Could you check a few things on this drawing? It's one solid part, dimensions in mm from its lowest x, y, z. A direction names the side the tool comes from. Give positions to 0.01 mm unless a question says otherwise; leave off trailing zeros. Write each loop counter-clockwise with the first axis right and the second up, starting at its lowest first coordinate (ties: lowest second). Pieces come first, ordered by that corner, then holes. Notation, with made-up numbers: M 26,8.25 L 69,8.25 A9 cw 69,13.25 Z; hole C 23.25,-32 d9. An arc over 180 degrees is marked long. Answer as CSV lines item,"result". Start each with the question number.
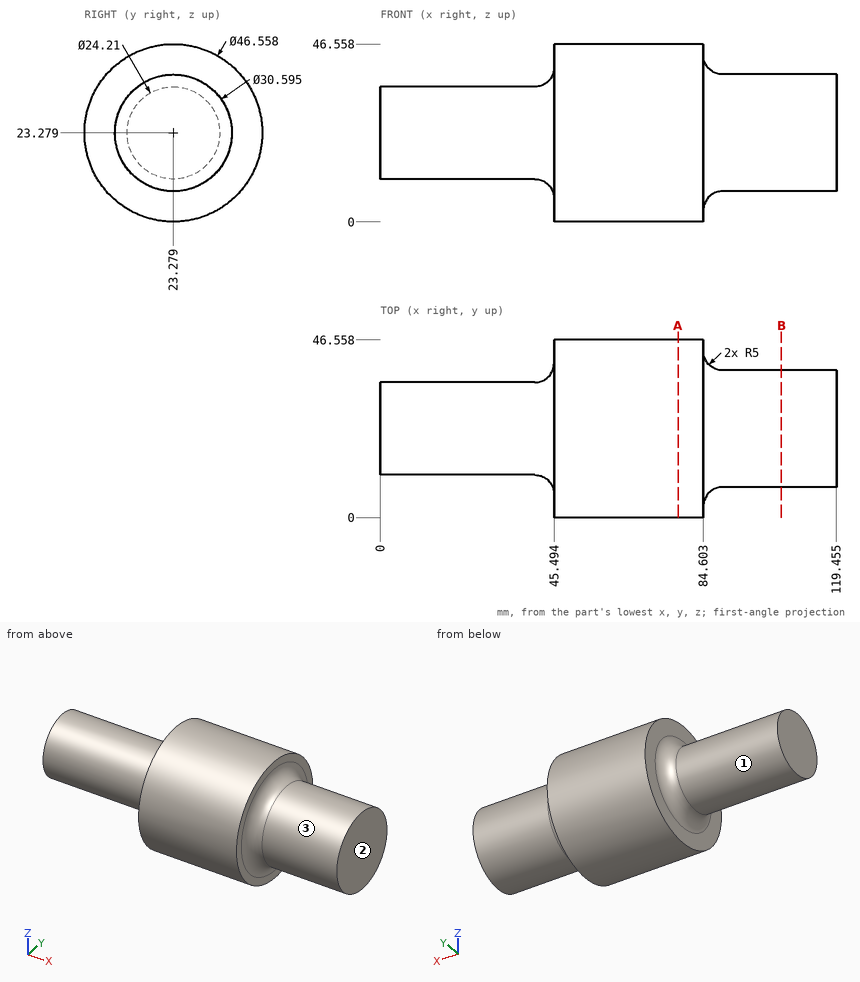
1) I want a section at B-B, the plane x = 105. Please give me the cut outline in (y, z) (1 decimal).
2) I'm going to push flat-ended pins straight in: P1, Ø8, axis at x = 61, z = 9.5, coming from the +Y side (1 decimal); P2, Ø2, axis at x = 29.5, y = 17, coming from the +Z side; P3, Ø10, axis at x = 49, z = 12.5, coming from the -Y side. Where does each tip first touch, or does it pass through?
3) On a 3-axis mill with a long thin cutter (end or side, diameter ignored), from which of +Z, -Z, +X, -X, +Y, -Y can I reach the whole of each face in a straight line? I mean the marked faces 1, 2 and 3. Say none if no direction works.
4) I want a section at A-A, the plane x = 78. Please give me the cut outline in (y, z).
5) I need wall thicknesses on L1, parallel to X at y = 8, z = 40; L2, parallel to Z at x = 91, y = 23.5 (1 decimal); L3, parallel to Z at x = 91.5, y = 33 (1 decimal). Which ranges of each line are inside material? Lowest first, please. Write a range as from..to.
Values found:
1,outline,"C 23.3,23.3 d30.6"
2,P1,"stops at y = 44.4"
2,P2,"stops at z = 34.17"
2,P3,"stops at y = 0.73"
3,face 1,"-X"
3,face 2,"+Z, -Z, +X, +Y, -Y"
3,face 3,"+X"
4,outline,"C 23.28,23.28 d46.56"
5,L1,"x = 45.49..84.6"
5,L2,"z = 8..38.6"
5,L3,"z = 11.5..35.1"
